```python
from build123d import *

# Parameters (mm, degrees)
F1_DEPTH = 38.1


with BuildPart() as f1:
    # F0 (on Front) → F1 (new body, symmetric)
    with BuildSketch(Plane.XZ):
        with BuildLine():
            Line((43.2224310935, 1.5943679027), (-23.4427358955, 0))
            Line((-23.4427358955, 0), (-65.5905306339, -3.9171427488))
            add(Edge.make_bspline(
                [(-65.5905306339, -3.9171427488), (-68.0041984956, -4.9276178366), (-72.229069768, -6.6963480077), (-72.7463312071, -11.6753389144), (-69.0538055852, -17.2946702596), (-59.6869487074, -20.5694560435), (-59.6583485603, -20.671416074)],
                knots=[0, 0, 0, 0, 0.2489109965, 0.4356924726, 0.6905546732, 0.9729684049, 0.9729684049, 0.9729684049, 0.9729684049], degree=3))
            Line((-59.6583485603, -20.671416074), (33.6398594081, -20.671416074))
            add(Edge.make_bspline(
                [(33.6398594081, -20.671416074), (35.8208168114, -18.40731191), (39.9250798829, -14.1465780249), (46.4031363616, -8.9319649582), (44.3428903861, -2.113717719), (43.2224310935, 1.5943679027)],
                knots=[0, 0, 0, 0, 0.3409172772, 0.6415596146, 1, 1, 1, 1], degree=3))
        make_face()
    extrude(amount=F1_DEPTH, both=True)


solid = f1.part
```
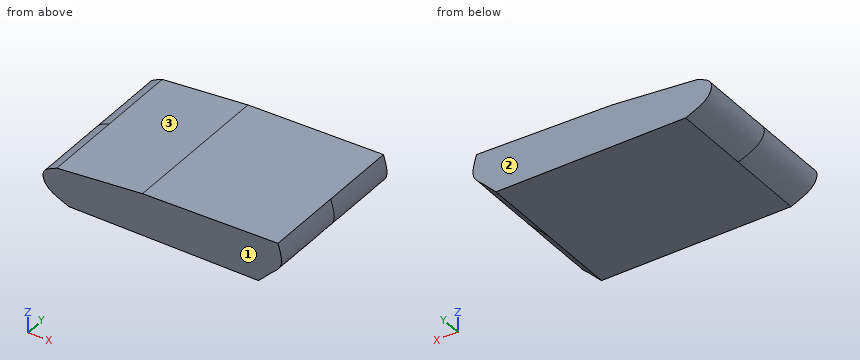
Work out the finished part from the listing and answer in its coordinate system (mm). Face numbers are marked on the shaded views. Give positions to 0.01 mm unless a question says otherwise; leave off trailing zeros. Write each loop counter-clockwise with the first axis right and the second up, starting at its lowest first coordinate (ties: lowest second). Pieces come first, ordered by that corner, then holes.
(1) The part is cut by section A-A on x = 18.5. Write down the section's boundary in (y, z).
Final values:
outline: (-38.1, -20.67) - (38.1, -20.67) - (38.1, 1) - (-38.1, 1) - close
(2) The mould has two halves that part along Y. Classify the marked faces 1, 2 and 3: pulls with the +Y half, pulls with the -Y half, needs draft (parallel to the pull), parting line crosses it, or undercut.
Final values:
face 1: pulls with the -Y half
face 2: pulls with the +Y half
face 3: needs draft
(3) Flat-ended cylindrical pins translate along their axes: pin 1 Ø3 at (y, z) = (29, -8.5) entering from -X; pin 2 Ø10 at (y, z) = (-7.5, -16) entering from -X; pin 3 Ø10 at (x, y) = (-51, -5.5) entering from +Z; pin 4 Ø12 at (x, y) = (-36, -28.5) entering from +Z. Find the tip coordinate at first contact, or state that the pin passes through.
Final values:
pin 1: stops at x = -72.39
pin 2: stops at x = -72.28
pin 3: stops at z = -2.1
pin 4: stops at z = -0.61
(4) Straight lines are drawn through the part: line 1 (Z direction, x = 27, y = -23); line 2 (X direction, y = 34, z = -6); line 3 (Z direction, x = 1, y = -8). For each, find the intervals that lie inside material, in ascending order.
Final values:
line 1: z = -20.67 to 1.21
line 2: x = -69.93 to 44.94
line 3: z = -20.67 to 0.58
(5) The part is cut by section B-B on x = -15.5. Write down the section's boundary in (y, z).
Final values:
outline: (-38.1, -20.67) - (38.1, -20.67) - (38.1, 0.19) - (-38.1, 0.19) - close
